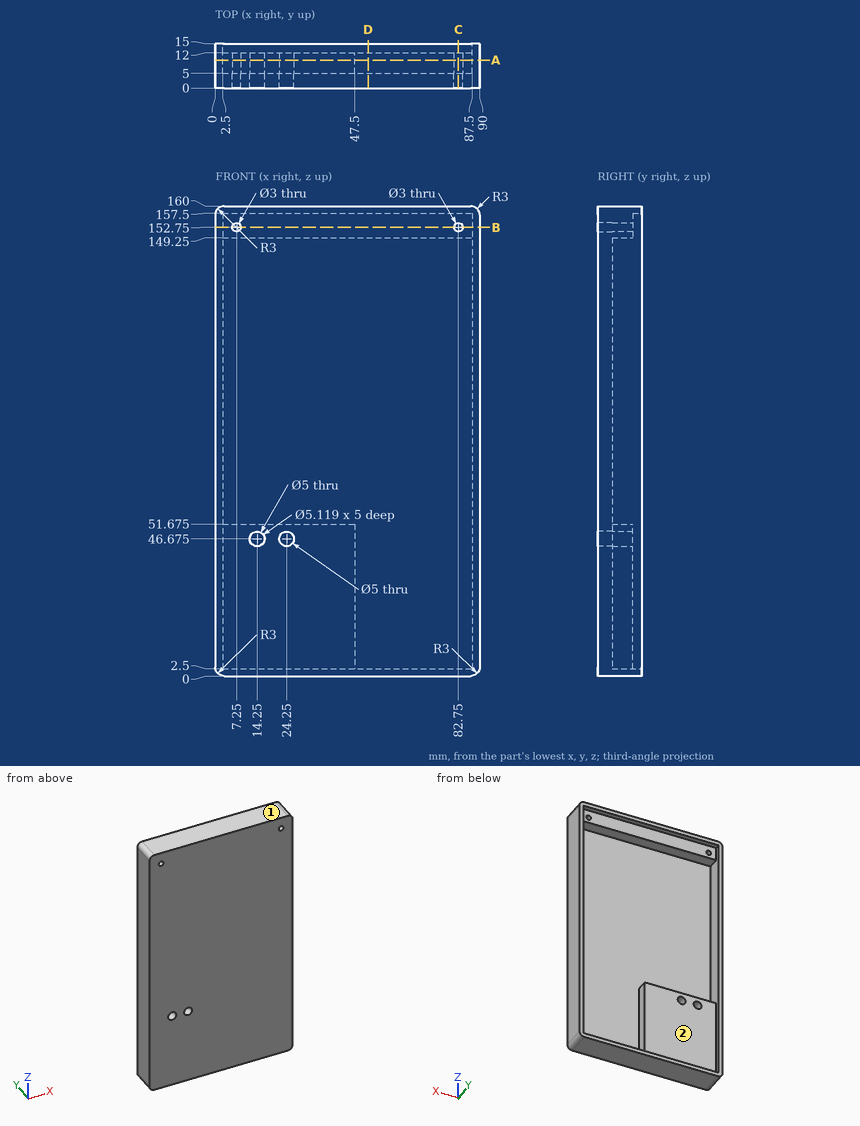
Print and shaded views of the part. All mm, measured from the part's lowest x, y and z. Coordinates: 2 decimals unless noted, no trailing zeros. Order: outer loops, then holes, each group sorted by start corner. A loop starts at its lowest first (then second) coordinate and runs counter-clockwise, first axis right, second up. Notation, with made-up numbers: M 67,82 L 122,82 A22 ccw 122,114 Z; hole C 50.5,-24 d7. An arc over 180 degrees is marked long. Answer as CSV lines item,"result".
1) Flat gauge pins, fed straight in: P1, Ø1, axis at x = 77.5, z = 103, coming from the +Y side; P2, Ø6.5, axis at x = 53.5, z = 153.5, coming from the +Y side. Where does each tip first touch, or does it go through?
Verdict:
P1,"y = 5"
P2,"y = 12"
2) Cut at A-A (y = 9.5). Give the number of separate pieces and of enclosed holes in the cut face, then the cut area to 3 significant figures.
Verdict:
separate pieces,"1"
enclosed holes,"5"
area,"4,080 mm2"
3) Cut at B-B (z = 152.75). List the corners of the cut face in (x, y).
Verdict:
outline,"M 0,0 L 5.75,0 L 5.75,12 L 2.5,12 L 2.5,15 L 0,15 Z; M 8.75,0 L 81.25,0 L 81.25,12 L 8.75,12 Z; M 84.25,0 L 90,0 L 90,15 L 87.5,15 L 87.5,12 L 84.25,12 Z"
4) Cut at C-C (x = 82.75). List the corners of the cut face in (y, z).
Verdict:
outline,"M 0,0 L 15,0 L 15,2.5 L 5,2.5 L 5,149.25 L 12,149.25 L 12,151.25 L 0,151.25 Z; M 0,154.25 L 12,154.25 L 12,157.5 L 15,157.5 L 15,160 L 0,160 Z"
5) Drill centre lines: L1, parallel to X at y = 1.85, z = 152.75; L2, parallel to Z at x = 82.75, y = 1.4; L3, parallel to Z at x = 33, y = 13. Where is each one in solid material? Low to high. Write a range as from..to.
Verdict:
L1,"0..5.75, 8.75..81.25, 84.25..90"
L2,"0..151.25, 154.25..160"
L3,"0..2.5, 157.5..160"
6) Cut at D-D (x = 52). List the corners of the cut face in (y, z).
Verdict:
outline,"M 0,0 L 15,0 L 15,2.5 L 5,2.5 L 5,149.25 L 12,149.25 L 12,157.5 L 15,157.5 L 15,160 L 0,160 Z"
7) Mould opens along X. For the marked faces 1 and 2 say: released by +X, released by -X, zero draft, split by the parting line, or undercut.
Verdict:
face 1,"zero draft"
face 2,"undercut"
